Source: three-view drawing plus pictorial views. Frame: mm from the lowest corner of the part. A direction names the side the tool comes from. Round coordinates to 2 decimals unless told otherwise and drop trailing zeros. Loops run counter-clockwise (first coordinate to the right, second up) from the corner with the lowest first, then second, coordinate; pieces in that order, holes last. Notation, with made-up numbers: (13, 25) -> (22, 25) arc R17 ccw to (22, 50) -> close; hole circle Ø10 at (77.25, 50.5). An arc over 180 degrees is marked (long way). Put each result on its own line as item: value. Start each with the question number.
1. Set-up query: the marked faces 1 and 2. Return all of +Z, -Z, +X, -X, +Y, -Y with unobstructed straight access to the full face (end or side cutting, diameter ignored); none if empty.
2. Material intervals for L1, parallel to Y at x = 2.25, z = 8.25; L2, parallel to X at y = 14.5, z = 1; L3, parallel to Z at x = 5.25, y = 15.25, sorted ascending.
3. Contact query for flat-ended pins moving along their axis: pin 1 (4 mm diameter, centred on x = 4.5, y = 2, fed in from +Z) (3 decimals); pin 2 (5 mm diameter, centred on y = 12.5, z = 5, fed in from -X) (3 decimals); pin 3 (2 mm diameter, centred on x = 6.5, y = 16, fed in from -Z). Output: stop coordinate, or through.
4. Cut plane A-A (y = 11.5). Return the cut outline in (x, z) (3 decimals), then the cut area to 3 significant figures.
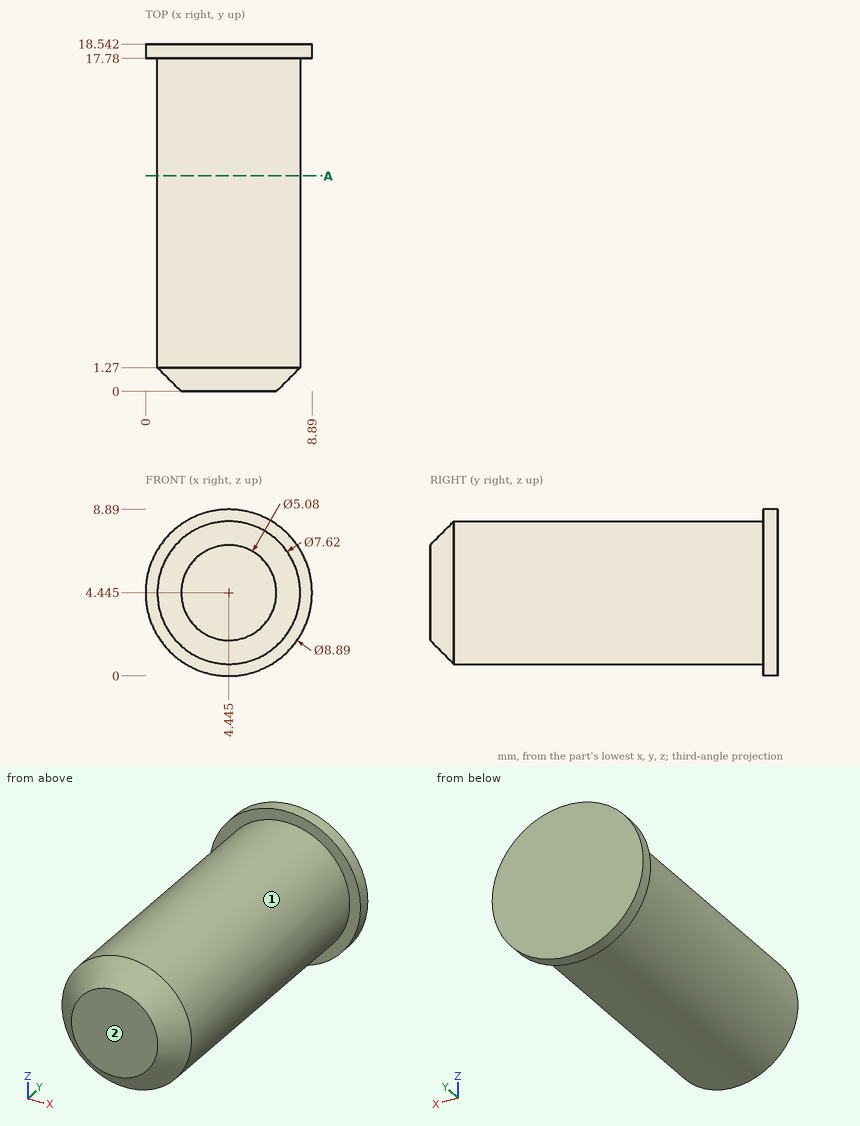
Solution:
1. face 1: -Y
1. face 2: +Z, -Z, +X, -X, -Y
2. L1: y = 17.78 to 18.54
2. L2: x = 2.82 to 6.07
2. L3: z = 0.72 to 8.17
3. pin 1: stops at z = 8.255
3. pin 2: stops at x = 0.635
3. pin 3: stops at z = 0.78
4. outline: circle Ø7.62 at (4.445, 4.445)
4. area: 45.6 mm^2
